The figure shows three views and two pictorial views of one solid part (mm, origin at its lowest corner). Answer the questions. Coordinates: 2 decimals unless noted, no trailing zeros. Write each loop counter-clockwise with the first axis right and the second up, starting at its lowest first coordinate (ties: lowest second). Pieces come first, ordered by that corner, then holes.
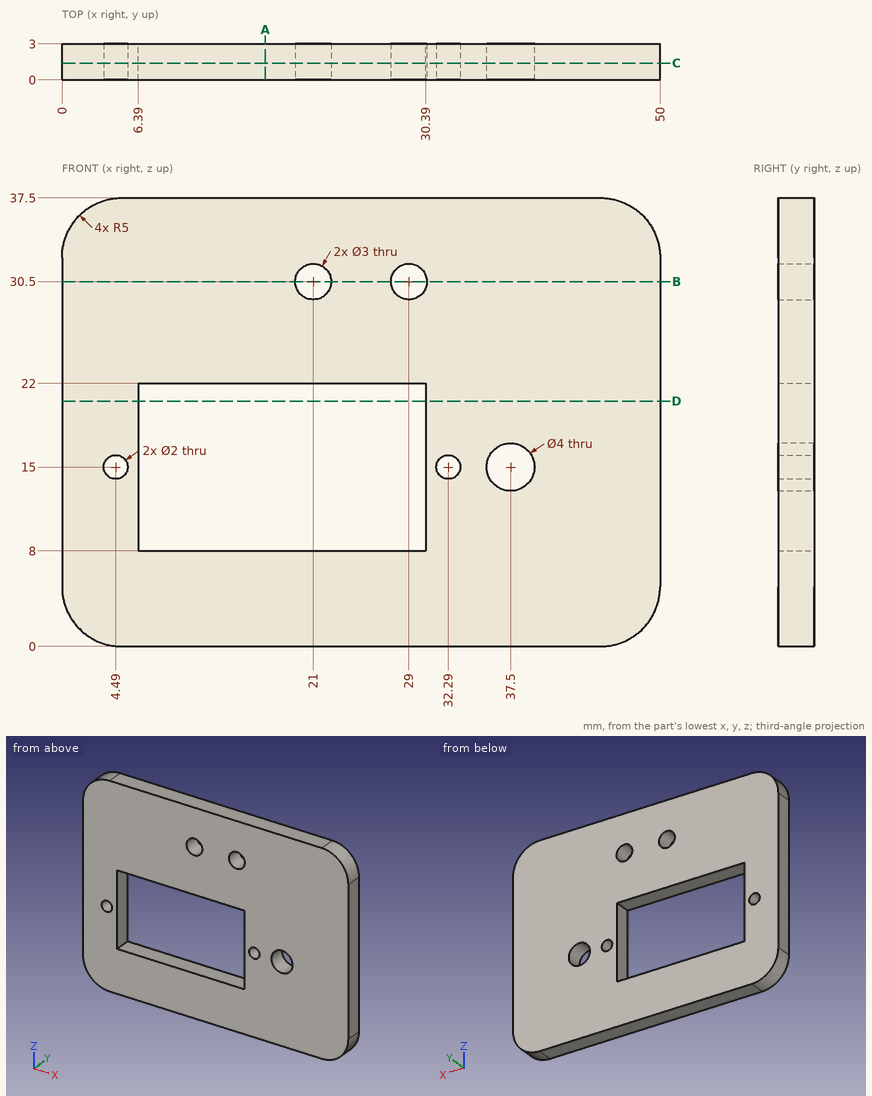
Q1. Given pin 1 (2.5 mm diameter, centred on x = 32.29, z = 15, fed in from -Y), flat-ended and moving along its own axis, determine where the tip first touches the part or whether it passes through.
Answers below:
pin 1: stops at y = 0
Q2. The part is cut by section A-A, the plane x = 17. Write down the section's boundary in (y, z), then the cut area to 3 significant figures.
Answers below:
outline: (0, 0) - (3, 0) - (3, 8) - (0, 8) - close; (0, 22) - (3, 22) - (3, 37.5) - (0, 37.5) - close
area: 70.5 mm2
Q3. Find the intervals of material crossed by probe 1 along X at (y, z) = (1.65, 15); probe 2 along Z at (x, y) = (21, 1.7); probe 3 along Z at (x, y) = (25.5, 2.35), in increasing order.
Answers below:
probe 1: x = 0 to 3.49, 5.49 to 6.39, 30.39 to 31.29, 33.29 to 35.5, 39.5 to 50
probe 2: z = 0 to 8, 22 to 29, 32 to 37.5
probe 3: z = 0 to 8, 22 to 37.5
Q4. The part is cut by section D-D, the plane z = 20.5. Write down the section's boundary in (x, y).
Answers below:
outline: (0, 0) - (6.39, 0) - (6.39, 3) - (0, 3) - close; (30.39, 0) - (50, 0) - (50, 3) - (30.39, 3) - close
Q5. The part is cut by section C-C, the plane y = 1.4. Write down the section's boundary in (x, z), then the cut area to 3 significant figures.
Answers below:
outline: (0, 5) arc R5 ccw to (5, 0) - (45, 0) arc R5 ccw to (50, 5) - (50, 32.5) arc R5 ccw to (45, 37.5) - (5, 37.5) arc R5 ccw to (0, 32.5) - close; hole circle Ø2 at (4.49, 15); hole (6.39, 8) - (30.39, 8) - (30.39, 22) - (6.39, 22) - close; hole circle Ø3 at (21, 30.5); hole circle Ø3 at (29, 30.5); hole circle Ø2 at (32.29, 15); hole circle Ø4 at (37.5, 15)
area: 1,480 mm2
Q6. The part is cut by section B-B, the plane z = 30.5. Write down the section's boundary in (x, y), then the cut area to 3 significant figures.
Answers below:
outline: (0, 0) - (19.5, 0) - (19.5, 3) - (0, 3) - close; (22.5, 0) - (27.5, 0) - (27.5, 3) - (22.5, 3) - close; (30.5, 0) - (50, 0) - (50, 3) - (30.5, 3) - close
area: 132 mm2
